For this review, take the finished solid that the model builds, in its own axes (mm). Coordinates: 2 decimals unless noted, no trailing zeros. Answer as a JSON object with one key per item and string values. Group by question number.
Item 1: Wall thickness on L1, parallel to Z at x = 127.5, y = -12.5; L2, parallel to Y at x = 102, z = -15.25; L3, parallel to Y at x = 213, z = -4: over which ranges is each line inside the solid? List them lowest first. Write a range as from..to.
Item 2: Add section A-A (x = 165.5). Count the separate pieces of the cut face and the enclosed holes in it, then the cut area to 3 significant figures.
Item 3: Insertion check: pin 1 (3 mm diameter, centred on x = 96.5, y = -7.5, fed in from -Z). The pin has a flat end and moves straight along its axis. Give the tip position at first contact, or say it passes through.
from build123d import *

# Parameters (mm, degrees)
SKETCH1_R           = 1.5
BOSS_EXTRUDE1_DEPTH = 300


with BuildPart() as part:
    # Sketch1 → Boss-Extrude1 (new body)
    with BuildSketch(Plane(origin=(-50, 0, 0), x_dir=(0, -1, 0), z_dir=(-1, 0, 0))):
        Polygon((5.2, -11.451471863), (3.751471863, -12.9), (1, -12.9), (1, -11.6), (0, -11.6), (0, -17.5), (5.9, -17.5), (5.9, -16.5), (4.6, -16.5), (4.6, -13.748528137), (6.048528137, -12.3), (8.951471863, -12.3), (10.4, -13.748528137), (10.4, -16.5), (9.1, -16.5), (9.1, -17.5), (15, -17.5), (15, -11.6), (14, -11.6), (14, -12.9), (11.248528137, -12.9), (9.8, -11.451471863), (9.8, -8.548528137), (11.248528137, -7.1), (14, -7.1), (14, -8.4), (15, -8.4), (15, -2.5), (9.1, -2.5), (9.1, -3.5), (10.4, -3.5), (10.4, -6.251471863), (8.951471863, -7.7), (6.048528137, -7.7), (4.6, -6.251471863), (4.6, -3.5), (5.9, -3.5), (5.9, -2.5), (0, -2.5), (0, -8.4), (1, -8.4), (1, -7.1), (3.751471863, -7.1), (5.2, -8.548528137), align=None)
        with Locations(Location((7.5, -10, 0), (0, 0, 270))):
            Circle(SKETCH1_R, mode=Mode.SUBTRACT)
        with Locations(Location((2.5, -5, 0), (0, 0, 270))):
            Circle(SKETCH1_R, mode=Mode.SUBTRACT)
        with Locations(Location((2.5, -15, 0), (0, 0, 270))):
            Circle(SKETCH1_R, mode=Mode.SUBTRACT)
        with Locations(Location((12.5, -5, 0), (0, 0, 270))):
            Circle(SKETCH1_R, mode=Mode.SUBTRACT)
        with Locations(Location((12.5, -15, 0), (0, 0, 270))):
            Circle(SKETCH1_R, mode=Mode.SUBTRACT)
    extrude(amount=-BOSS_EXTRUDE1_DEPTH)


solid = part.part
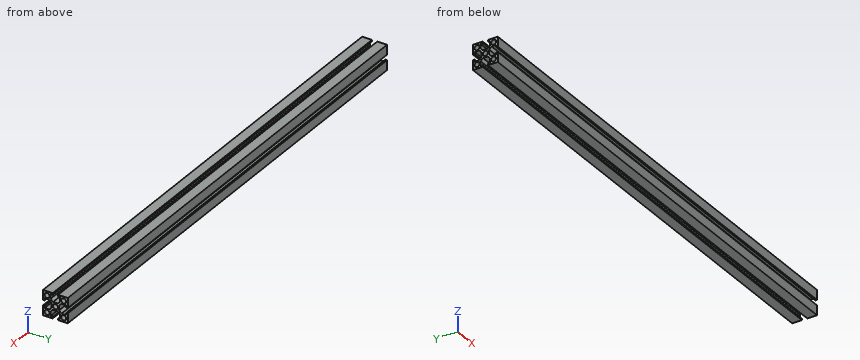
From the geometry:
{
 "1": {"L1": "z = -17.5..-16.5, -13.5..-12.9, -7.1..-6.5, -3.5..-2.5", "L2": "y = -15..-13.98, -11.02..-10.4, -4.6..-3.98, -1.02..0", "L3": "y = -15..-13.62, -11.38..-10.4, -4.6..-3.62, -1.38..0"},
 "2": {"separate pieces": "1", "enclosed holes": "5", "area": "87.8 mm²"},
 "3": {"pin 1": "stops at z = -12.35"}
}
